Can you work these out from the model? Positions are in its coordinate system, mm. Face numbers are marked on the shaded views. A direction names the side the tool comes from. Coordinates: 2 decimals unless noted, no trailing zeros. Order: outer loops, then holes, each group sorted by start corner. A loop starts at its lowest first (then second) coordinate and runs counter-clockwise, first axis right, second up. Notation, with made-up numbers: (36.25, -7) -> (53.25, -7) arc R9 cw to (53.25, 4) -> close; hole circle Ø1 at (59.5, 14). An arc over 180 degrees is marked (long way). Return JSON: item names as keys, results as strings. Group by question number.
1) Thinking about a two-plate mould opening in X: for the marked faces 1 and 2, which applies, +X half, -X half, draft (parallel to the pull), parting line (faces both ways), or undercut?
2) If we section it at B-B, the plane x = 62: Please give me the cut outline in (y, z), then the cut area to 3 significant figures.
3) If we section it at D-D, the plane x = -11.5: Please give me the cut outline in (y, z), then the cut area to 3 significant figures.
4) For the marked faces 3 and 4, which set-ups out of +Z, -Z, +X, -X, +Y, -Y let a thin tool reach every point of the face, with its end or its side?
5) If I drill on probe 1 along Y at (x, z) = (85.5, -1.8); probe 2 along Y at (x, z) = (-21, -2); probe 3 along Y at (x, z) = (43, -2), over which ranges is the centre line in solid material (lowest first)? Write a range as from..to.
6) If we section it at A-A, the plane z = -2.5: Please give me the cut outline in (x, y) (3 decimals).
7) If we section it at C-C, the plane y = -9: Please give me the cut outline in (x, z).
8) For pin 1 (3 mm diameter, centred on y = 27.5, z = -2.5, fed in from +X); pin 2 (2 mm diameter, centred on x = 3, z = -4, fed in from -Y); pin 3 (8 mm diameter, centred on x = -64.5, y = -15.5, fed in from -Z), each with a flat end and sliding along its axis, tell me the tip position at first contact or that it passes through.
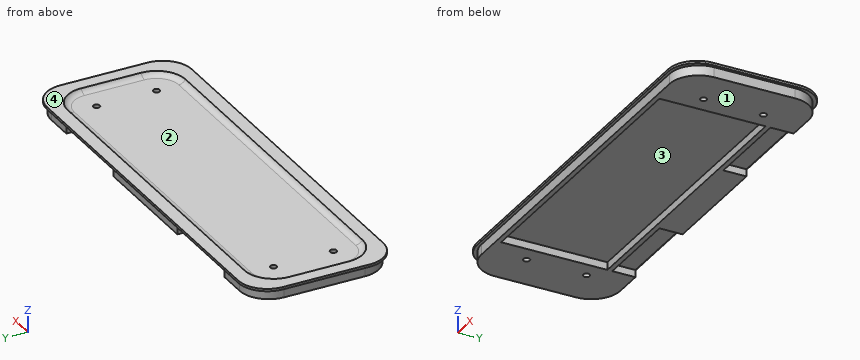
from build123d import *

# Parameters (mm, degrees)
F0_W          = 215
F0_H          = 75
F1_DEPTH      = 1.25
F2_R          = 15
F3_W          = 212
F3_H          = 72
F4_DEPTH      = 5.25
F5_T1_DEPTH   = 42.75
F7_W          = 201
F7_H          = 61
F8_DEPTH      = 2
F9_R          = 15
F10_T1_DEPTH  = 31
F10_T3_DEPTH  = 171
F10_T6_ANGLE  = 90
F10_T8_ANGLE  = 90
F10_T10_ANGLE = 90
F10_T12_ANGLE = 90
F11_W         = 45.625
F11_H         = 3.75
F12_DEPTH     = 12
F13_W         = 153
F13_H         = 55
F14_DEPTH     = 4
F16_D         = 3.4


# Not quite as in the source:
# - a fillet or chamfer that OpenCascade refuses, or shapes differently, is made with other operations: its cross-section is extruded or revolved along the edge and cut away or added


with BuildPart() as f1:
    # F0 (on Top) → F1 (new body)
    with BuildSketch(Plane.XY):
        Rectangle(F0_W, F0_H)
    extrude(amount=F1_DEPTH)

    # F2
    f2_edges = [f1.edges().sort_by_distance(p)[0] for p in [
        (107.5, -37.5, 0.625),
        (107.5, 37.5, 0.625),
        (-107.5, 37.5, 0.625),
        (-107.5, -37.5, 0.625),
    ]]
    fillet(f2_edges, radius=F2_R)

    # F3 (on face) → F4 (join)
    with BuildSketch(Plane(origin=(0, 0, 0), x_dir=(1, 0, 0), z_dir=(0, 0, -1))):
        Rectangle(F3_W, F3_H)
    extrude(amount=F4_DEPTH)

    # F5: fillet of radius 15 on 4 edges, made by hand

    # F5_s2 → F5_t1 (cut)
    with BuildSketch(Plane.XY.offset(-42.75)):
        with BuildLine():
            ThreePointArc((-106, -21), (-101.6066017178, -31.6066017178), (-91, -36))
            Line((-91, -36), (-106, -36))
            Line((-106, -36), (-106, -21))
        make_face()
        with BuildLine():
            ThreePointArc((-91, 36), (-101.6066017178, 31.6066017178), (-106, 21))
            Line((-106, 21), (-106, 36))
            Line((-106, 36), (-91, 36))
        make_face()
        with BuildLine():
            ThreePointArc((91, 36), (101.6066017178, 31.6066017178), (106, 21))
            Line((106, 21), (106, 36))
            Line((106, 36), (91, 36))
        make_face()
        with BuildLine():
            ThreePointArc((106, -21), (101.6066017178, -31.6066017178), (91, -36))
            Line((91, -36), (106, -36))
            Line((106, -36), (106, -21))
        make_face()
    extrude(amount=F5_T1_DEPTH, mode=Mode.SUBTRACT)

    # F7 (on face) → F8 (cut)
    with BuildSketch(Plane.XY.offset(1.25)):
        Rectangle(F7_W, F7_H)
    extrude(amount=-F8_DEPTH, mode=Mode.SUBTRACT)

    # F9
    f9_edges = [f1.edges().sort_by_distance(p)[0] for p in [
        (-100.5, 30.5, 0.25),
        (-100.5, -30.5, 0.25),
        (100.5, 30.5, 0.25),
        (100.5, -30.5, 0.25),
    ]]
    fillet(f9_edges, radius=F9_R)

    # F10: fillet of radius 4 on 1 edges, made by hand

    # F10_s2 → F10_t1 (join)
    with BuildSketch(Plane.XZ.offset(-15.5)):
        with BuildLine():
            ThreePointArc((-100.5, 1.25), (-99.0358983849, -0.2141016151), (-97.0358983849, -0.75))
            Line((-97.0358983849, -0.75), (-100.5, -0.75))
            Line((-100.5, -0.75), (-100.5, 1.25))
        make_face()
        with BuildLine():
            ThreePointArc((100.5, 1.25), (99.0358983849, -0.2141016151), (97.0358983849, -0.75))
            Line((97.0358983849, -0.75), (100.5, -0.75))
            Line((100.5, -0.75), (100.5, 1.25))
        make_face()
    extrude(amount=F10_T1_DEPTH)

    # F10_s4 → F10_t3 (join)
    with BuildSketch(Plane.YZ.offset(-85.5)):
        with BuildLine():
            ThreePointArc((-30.5, 1.25), (-29.0358983849, -0.2141016151), (-27.0358983849, -0.75))
            Line((-27.0358983849, -0.75), (-30.5, -0.75))
            Line((-30.5, -0.75), (-30.5, 1.25))
        make_face()
        with BuildLine():
            ThreePointArc((30.5, 1.25), (29.0358983849, -0.2141016151), (27.0358983849, -0.75))
            Line((27.0358983849, -0.75), (30.5, -0.75))
            Line((30.5, -0.75), (30.5, 1.25))
        make_face()
    extrude(amount=F10_T3_DEPTH)

    # F10_s5 → F10_t6 (revolve)
    with BuildSketch(Plane.YZ.offset(-85.5)):
        with BuildLine():
            ThreePointArc((30.5, 1.25), (29.0358983849, -0.2141016151), (27.0358983849, -0.75))
            Line((27.0358983849, -0.75), (30.5, -0.75))
            Line((30.5, -0.75), (30.5, 1.25))
        make_face()
    revolve(axis=Axis((-85.5, 15.5, -0.75), (0, 0, 1)), revolution_arc=F10_T6_ANGLE)

    # F10_s7 → F10_t8 (revolve)
    with BuildSketch(Plane.XZ.offset(15.5)):
        with BuildLine():
            ThreePointArc((-100.5, 1.25), (-99.0358983849, -0.2141016151), (-97.0358983849, -0.75))
            Line((-97.0358983849, -0.75), (-100.5, -0.75))
            Line((-100.5, -0.75), (-100.5, 1.25))
        make_face()
    revolve(axis=Axis((-85.5, -15.5, -0.75), (0, 0, 1)), revolution_arc=F10_T8_ANGLE)

    # F10_s9 → F10_t10 (revolve)
    with BuildSketch(Plane.YZ.offset(85.5)):
        with BuildLine():
            ThreePointArc((-30.5, 1.25), (-29.0358983849, -0.2141016151), (-27.0358983849, -0.75))
            Line((-27.0358983849, -0.75), (-30.5, -0.75))
            Line((-30.5, -0.75), (-30.5, 1.25))
        make_face()
    revolve(axis=Axis((85.5, -15.5, -0.75), (0, 0, 1)), revolution_arc=F10_T10_ANGLE)

    # F10_s11 → F10_t12 (revolve)
    with BuildSketch(Plane.YZ.offset(85.5)):
        with BuildLine():
            ThreePointArc((30.5, 1.25), (29.0358983849, -0.2141016151), (27.0358983849, -0.75))
            Line((27.0358983849, -0.75), (30.5, -0.75))
            Line((30.5, -0.75), (30.5, 1.25))
        make_face()
    revolve(axis=Axis((85.5, 15.5, -0.75), (0, 0, -1)), revolution_arc=F10_T12_ANGLE)

    # F11 (on face) → F12 (cut)
    with BuildSketch(Plane(origin=(0, 36, 0), x_dir=(-1, 0, 0), z_dir=(0, 1, 0))):
        with Locations((-53.6875, -3.375)):
            Rectangle(F11_W, F11_H)
        with Locations((53.6875, -3.375)):
            Rectangle(F11_W, F11_H)
    extrude(amount=-F12_DEPTH, mode=Mode.SUBTRACT)

    # F13 (on face) → F14 (cut)
    with BuildSketch(Plane(origin=(0, 0, -5.25), x_dir=(1, 0, 0), z_dir=(0, 0, -1))):
        with Locations((0, 6)):
            Rectangle(F13_W, F13_H)
    extrude(amount=-F14_DEPTH, mode=Mode.SUBTRACT)

    # F16 (through all)
    with Locations(Plane.XY.offset(1.25)):
        with Locations((-85.5, 15.5), (-85.5, -15.5), (85.5, 15.5), (85.5, -15.5)):
            Hole(F16_D / 2)


solid = f1.part
Result sheet:
{
 "1": {"face 1": "draft", "face 2": "undercut"},
 "2": {"outline": "(-37.5, 0) -> (-36, 0) -> (-36, -5.25) -> (-33.5, -5.25) -> (-33.5, -1.25) -> (21.5, -1.25) -> (21.5, -5.25) -> (24, -5.25) -> (24, -1.5) -> (36, -1.5) -> (36, 0) -> (37.5, 0) -> (37.5, 1.25) -> (30.5, 1.25) arc R4 cw to (27.04, -0.75) -> (-27.04, -0.75) arc R4 cw to (-30.5, 1.25) -> (-37.5, 1.25) -> close", "area": "88.8 mm2"},
 "3": {"outline": "(-37.5, 0) -> (-36, 0) -> (-36, -5.25) -> (-33.5, -5.25) -> (-33.5, -1.25) -> (21.5, -1.25) -> (21.5, -5.25) -> (36, -5.25) -> (36, 0) -> (37.5, 0) -> (37.5, 1.25) -> (30.5, 1.25) arc R4 cw to (27.04, -0.75) -> (-27.04, -0.75) arc R4 cw to (-30.5, 1.25) -> (-37.5, 1.25) -> close", "area": "134 mm2"},
 "4": {"face 3": "-Z", "face 4": "+Z, +X, -X, +Y, -Y"},
 "5": {"probe 1": "y = -36..-17.2, -13.8..13.8, 17.2..36", "probe 2": "y = -36..-33.5, 21.5..36", "probe 3": "y = -36..-33.5, 21.5..24"},
 "6": {"outline": "(-106, -21) arc R15 ccw to (-91, -36) -> (91, -36) arc R15 ccw to (106, -21) -> (106, 21) arc R15 ccw to (91, 36) -> (76.5, 36) -> (76.5, 24) -> (30.875, 24) -> (30.875, 36) -> (-30.875, 36) -> (-30.875, 24) -> (-76.5, 24) -> (-76.5, 36) -> (-91, 36) arc R15 ccw to (-106, 21) -> close; hole circle Ø3.4 at (-85.5, -15.5); hole circle Ø3.4 at (-85.5, 15.5); hole (-76.5, -33.5) -> (76.5, -33.5) -> (76.5, 21.5) -> (-76.5, 21.5) -> close; hole circle Ø3.4 at (85.5, -15.5); hole circle Ø3.4 at (85.5, 15.5)"},
 "7": {"outline": "(-107.5, 0) -> (-106, 0) -> (-106, -5.25) -> (-76.5, -5.25) -> (-76.5, -1.25) -> (76.5, -1.25) -> (76.5, -5.25) -> (106, -5.25) -> (106, 0) -> (107.5, 0) -> (107.5, 1.25) -> (100.5, 1.25) arc R4 cw to (97.04, -0.75) -> (-97.04, -0.75) arc R4 cw to (-100.5, 1.25) -> (-107.5, 1.25) -> close"},
 "8": {"pin 1": "stops at x = 105.14", "pin 2": "stops at y = -36", "pin 3": "stops at z = -1.25"}
}
